from build123d import *

# Parameters (mm, degrees)
F0_R     = 12.7
F1_DEPTH = 88.9
F2_R     = 12.7
F3_DEPTH = 12.7
F4_R     = 1.5875
F5_R     = 6.35


with BuildPart() as f1:
    # F0 (on Top) → F1 (new body)
    with BuildSketch(Plane.XY):
        Circle(F0_R)
        with BuildLine():
            ThreePointArc((-2.9826358368, 1.0883512598), (-1.866218176, 2.5686289571), (-0.1133983961, 3.1729742835))
            Line((-0.1133983961, 3.1729742835), (0, 2.9765625))
            Line((0, 2.9765625), (0.1133983961, 3.1729742835))
            ThreePointArc((0.1133983961, 3.1729742835), (1.866218176, 2.5686289571), (2.9826358368, 1.0883512598))
            Line((2.9826358368, 1.0883512598), (2.8308791618, 0.9198083973))
            Line((2.8308791618, 0.9198083973), (3.0527198999, 0.8726546928))
            ThreePointArc((3.0527198999, 0.8726546928), (3.0196044392, -0.9811289571), (1.9567687193, -2.5003362132))
            Line((1.9567687193, -2.5003362132), (1.74957954, -2.4080896473))
            Line((1.74957954, -2.4080896473), (1.7732862602, -2.6336440229))
            ThreePointArc((1.7732862602, -2.6336440229), (0, -3.175), (-1.7732862602, -2.6336440229))
            Line((-1.7732862602, -2.6336440229), (-1.74957954, -2.4080896473))
            Line((-1.74957954, -2.4080896473), (-1.9567687193, -2.5003362132))
            ThreePointArc((-1.9567687193, -2.5003362132), (-3.0196044392, -0.9811289571), (-3.0527198999, 0.8726546928))
            Line((-3.0527198999, 0.8726546928), (-2.8308791618, 0.9198083973))
            Line((-2.8308791618, 0.9198083973), (-2.9826358368, 1.0883512598))
        make_face(mode=Mode.SUBTRACT)
    extrude(amount=F1_DEPTH)

    # F2 (on face) → F3 (join)
    with BuildSketch(Plane.XY.offset(88.9)):
        Circle(F2_R)
        with BuildLine():
            Line((-2.8308791618, 0.9198083973), (-2.9826358368, 1.0883512598))
            ThreePointArc((-2.9826358368, 1.0883512598), (-1.866218176, 2.5686289571), (-0.1133983961, 3.1729742835))
            Line((-0.1133983961, 3.1729742835), (0, 2.9765625))
            Line((0, 2.9765625), (0.1133983961, 3.1729742835))
            ThreePointArc((0.1133983961, 3.1729742835), (1.866218176, 2.5686289571), (2.9826358368, 1.0883512598))
            Line((2.9826358368, 1.0883512598), (2.8308791618, 0.9198083973))
            Line((2.8308791618, 0.9198083973), (3.0527198999, 0.8726546928))
            ThreePointArc((3.0527198999, 0.8726546928), (3.0196044392, -0.9811289571), (1.9567687193, -2.5003362132))
            Line((1.9567687193, -2.5003362132), (1.74957954, -2.4080896473))
            Line((1.74957954, -2.4080896473), (1.7732862602, -2.6336440229))
            ThreePointArc((1.7732862602, -2.6336440229), (0, -3.175), (-1.7732862602, -2.6336440229))
            Line((-1.7732862602, -2.6336440229), (-1.74957954, -2.4080896473))
            Line((-1.74957954, -2.4080896473), (-1.9567687193, -2.5003362132))
            ThreePointArc((-1.9567687193, -2.5003362132), (-3.0196044392, -0.9811289571), (-3.0527198999, 0.8726546928))
            Line((-3.0527198999, 0.8726546928), (-2.8308791618, 0.9198083973))
        make_face(mode=Mode.SUBTRACT)
        with BuildLine():
            ThreePointArc((-0.1133983961, 3.1729742835), (-1.866218176, 2.5686289571), (-2.9826358368, 1.0883512598))
            Line((-2.9826358368, 1.0883512598), (-2.8308791618, 0.9198083973))
            Line((-2.8308791618, 0.9198083973), (-3.0527198999, 0.8726546928))
            ThreePointArc((-3.0527198999, 0.8726546928), (-3.0196044392, -0.9811289571), (-1.9567687193, -2.5003362132))
            Line((-1.9567687193, -2.5003362132), (-1.74957954, -2.4080896473))
            Line((-1.74957954, -2.4080896473), (-1.7732862602, -2.6336440229))
            ThreePointArc((-1.7732862602, -2.6336440229), (0, -3.175), (1.7732862602, -2.6336440229))
            Line((1.7732862602, -2.6336440229), (1.74957954, -2.4080896473))
            Line((1.74957954, -2.4080896473), (1.9567687193, -2.5003362132))
            ThreePointArc((1.9567687193, -2.5003362132), (3.0196044392, -0.9811289571), (3.0527198999, 0.8726546928))
            Line((3.0527198999, 0.8726546928), (2.8308791618, 0.9198083973))
            Line((2.8308791618, 0.9198083973), (2.9826358368, 1.0883512598))
            ThreePointArc((2.9826358368, 1.0883512598), (1.866218176, 2.5686289571), (0.1133983961, 3.1729742835))
            Line((0.1133983961, 3.1729742835), (0, 2.9765625))
            Line((0, 2.9765625), (-0.1133983961, 3.1729742835))
        make_face()
    extrude(amount=F3_DEPTH)

    # F4
    f4_edges = [f1.edges().sort_by_distance(p)[0] for p in [
        (-12.7, 0, 101.6),
    ]]
    fillet(f4_edges, radius=F4_R)

    # F5
    f5_edges = [f1.edges().sort_by_distance(p)[0] for p in [
        (-12.7, 0, 0),
    ]]
    fillet(f5_edges, radius=F5_R)


solid = f1.part
Here's how the part is built. I have some questions about the finished solid (model axes, mm). A direction names the side the tool comes from. Give positions to 0.01 mm unless a question says otherwise; leave off trailing zeros. Loops run counter-clockwise (first coordinate to the right, second up) from the corner with the lowest first, then second, coordinate; pieces in that order, holes last. Notation, with made-up numbers: (60.25, 50.25) -> (79.25, 50.25) arc R31 cw to (79.25, 74.25) -> close; hole circle Ø11 at (20.5, -8.75). An arc over 180 degrees is marked (long way). Answer as a JSON object with one key per item and string values. Group by question number.
Item 1: Imagine slicing it at A-A on z = 26. Write out the boundary of the cut face in (x, y) (3 decimals), then the cut area to 3 significant figures.
Item 2: Imagine slicing it at B-B on z = 92.5. Write out the boundary of the cut face in (x, y).
Item 3: On a 3-axis mill with a long thin cutter (end or side, diameter ignored), from which of +Z, -Z, +X, -X, +Y, -Y can I reach the whole of each face in a straight line? I mean faces 4 (the flat face through (-2, 3, 0)), 5 (the cylindrical face through (1.845, 2.584, 43.828)). Say none if no direction works.
Item 4: Will these pins go through, and if not, where does the flat tip stop? pin 1 (8 mm diameter, centred on x = -9, z = 67.5, fed in from -Y); pin 2 (8 mm diameter, centred on x = -1.5, z = 55.5, fed in from +Y); pin 3 (10 mm diameter, centred on x = -7, z = 13.5, fed in from +Y); pin 4 (6 mm diameter, centred on x = 9, z = 24.5, fed in from +Y).
Item 5: I need wall thicknesses on L1, parallel to X at y = 2.25, z = 15.5; L2, parallel to Y at x = 2, z = 27; L3, parallel to X at y = 0.5, z = 16. Which ranges of each line are inside material? Lowest first, please.
Item 6: Thinking about a two-plate mould opening in Y: for faces 1 (the cylindrical face through (-2.75, -12.4, 52.53)), 2 (the flat face through (0, 0, 88.9)), 3 (the flat face through (0, 0, 101.6)), which applies, pulls with the +Y half, pulls with the -Y half, needs draft (parallel to the pull), parting line crosses it, or undercut?
Answer list:
{
 "1": {"outline": "circle Ø25.4 at (0, 0); hole (-3.053, 0.873) arc R3.175 ccw to (-1.957, -2.5) -> (-1.75, -2.408) -> (-1.773, -2.634) arc R3.175 ccw to (1.773, -2.634) -> (1.75, -2.408) -> (1.957, -2.5) arc R3.175 ccw to (3.053, 0.873) -> (2.831, 0.92) -> (2.983, 1.088) arc R3.175 ccw to (0.113, 3.173) -> (0, 2.977) -> (-0.113, 3.173) arc R3.175 ccw to (-2.983, 1.088) -> (-2.831, 0.92) -> close", "area": "475 mm2"},
 "2": {"outline": "circle Ø25.4 at (0, 0)"},
 "3": {"face 4": "-Z, +X, -X, +Y, -Y", "face 5": "-Z"},
 "4": {"pin 1": "stops at y = -11.67", "pin 2": "stops at y = 12.7", "pin 3": "stops at y = 12.54", "pin 4": "stops at y = 11.19"},
 "5": {"L1": "x = -12.5 to -2.24, 2.24 to 12.5", "L2": "y = -12.54 to -2.47, 2.47 to 12.54", "L3": "x = -12.69 to -3.14, 3.14 to 12.69"},
 "6": {"face 1": "parting line crosses it", "face 2": "undercut", "face 3": "needs draft"}
}
